from build123d import *

# Parameters (mm, degrees)
SKETCH1_R           = 13.000723037
SKETCH1_R_2         = 5.55
SKETCH1_R_3         = 0.8
PLACA_CABEZAL_DEPTH = 4
SKETCH2_W           = 7.5
SKETCH2_H           = 9
PATA_AL_HUESO_DEPTH = 4


with BuildPart() as part:
    # Sketch1 → Placa_cabezal (new body)
    with BuildSketch(Plane(origin=(0, -2, 0), x_dir=(1, 0, 0), z_dir=(0, 1, 0))):
        with Locations(Location((0, 0, 0), (0, 0, 270))):
            Circle(SKETCH1_R)
        with Locations(Location((0, 6.5, 0), (0, 0, 270))):
            Circle(SKETCH1_R_2, mode=Mode.SUBTRACT)
        with Locations(Location((-5.63, -3.25, 0), (0, 0, 270))):
            Circle(SKETCH1_R_2, mode=Mode.SUBTRACT)
        with Locations(Location((5.63, -3.25, 0), (0, 0, 270))):
            Circle(SKETCH1_R_2, mode=Mode.SUBTRACT)
        with Locations(Location((0, 0, 0), (0, 0, 270))):
            Circle(SKETCH1_R_3, mode=Mode.SUBTRACT)
    extrude(amount=PLACA_CABEZAL_DEPTH)

    # Sketch2 → Pata_al_hueso (add)
    with BuildSketch(Plane(origin=(0, -2, 0), x_dir=(1, 0, 0), z_dir=(0, 1, 0))):
        with Locations((-15.250723037, 0)):
            Rectangle(SKETCH2_W, SKETCH2_H)
    extrude(amount=PATA_AL_HUESO_DEPTH)


solid = part.part
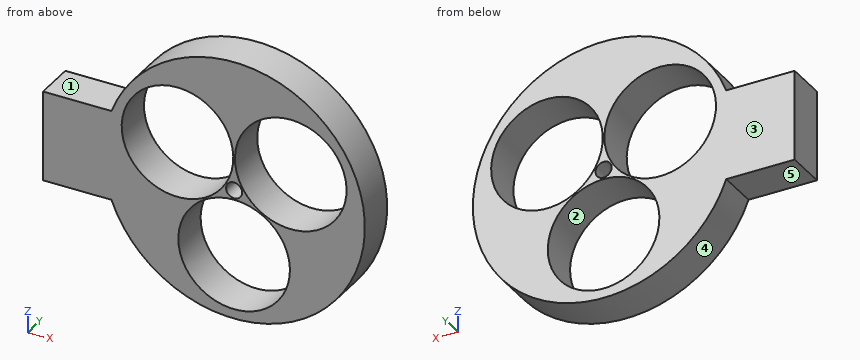
Here's how the part is built. I have some questions about the finished solid (model axes, mm). Face numbers are marked on the shaded views. A direction names the side the tool comes from. Round coordinates to 2 decimals unless told otherwise and drop trailing zeros. Order: outer loops, then holes, each group sorted by start corner. A loop starts at its lowest first (then second) coordinate and runs counter-clockwise, first axis right, second up. Notation, with made-up numbers: (62.5, -26.75) -> (88.5, -26.75) arc R17 ccw to (88.5, -4.75) -> close; hole circle Ø6 at (69.5, -1.75). An arc over 180 degrees is marked (long way). Return JSON: item names as keys, results as strings.
Q1. I need wall thicknesses on line 1 along X through (y, z) = (-0.6, 4); line 2 along X through (y, z) = (-0.9, 3.25); line 3 along Z through (x, y) = (-4.5, -1.2). Which ranges of each line are inside material? Lowest first, please. Write a range as from..to.
Filled sheet:
{"line 1": "x = -19..-11.13, -0.13..0.13, 11.13..12.37", "line 2": "x = -19..-11.18, -0.08..0.08, 11.18..12.59", "line 3": "z = -12.2..-9.75, -3.25..-2.18, 8.68..12.2"}
Q2. If we section it at C-C on y = -1.6: List the corners of the cut face in (x, z) for me.
Filled sheet:
{"outline": "(-19, -4.5) -> (-12.2, -4.5) arc R13 ccw (long way) to (-12.2, 4.5) -> (-19, 4.5) -> close; hole circle Ø11.1 at (-5.63, 3.25); hole circle Ø11.1 at (0, -6.5); hole circle Ø1.6 at (0, 0); hole circle Ø11.1 at (5.63, 3.25)"}
Q3. If we mould it in two halves opening along Z, with no side actions, what happens to the marked faces 1, 2 and 3? For each: released by +Z, released by -Z, zero draft, split by the parting line, or undercut.
Filled sheet:
{"face 1": "released by +Z", "face 2": "undercut", "face 3": "zero draft"}
Q4. If we section it at B-B on x = -2: List the corners of the cut face in (y, z) for me.
Filled sheet:
{"outline": "(-2, -12.85) -> (2, -12.85) -> (2, -11.68) -> (-2, -11.68) -> close; (-2, -1.32) -> (2, -1.32) -> (2, -0.95) -> (-2, -0.95) -> close; (-2, 7.45) -> (2, 7.45) -> (2, 12.85) -> (-2, 12.85) -> close"}
Q5. Which directions (+Z, -Z, +X, -X, +Y, -Y) give clear straight access to the entire face, cutting with the end or side of a thin tool? Please do the marked faces 4 and 5.
Filled sheet:
{"face 4": "+Y, -Y", "face 5": "-Z, -X, +Y, -Y"}
Q6. If we section it at D-D on z = -7: List the corners of the cut face in (x, y) for me, plus the area to 3 significant figures.
Filled sheet:
{"outline": "(-10.96, -2) -> (-5.53, -2) -> (-5.53, 2) -> (-10.96, 2) -> close; (5.53, -2) -> (10.96, -2) -> (10.96, 2) -> (5.53, 2) -> close", "area": "43.4 mm^2"}
Q7. If we section it at A-A on z = 2: List the corners of the cut face in (x, y) for me, plus the area to 3 significant figures.
Filled sheet:
{"outline": "(-19, -2) -> (-11.04, -2) -> (-11.04, 2) -> (-19, 2) -> close; (-0.22, -2) -> (0.22, -2) -> (0.22, 2) -> (-0.22, 2) -> close; (11.04, -2) -> (12.85, -2) -> (12.85, 2) -> (11.04, 2) -> close", "area": "40.9 mm^2"}
Q8. For pin 1 Ø1 at (y, z) = (-1.5, 2) entering from +X; pin 2 Ø1.2 at (x, y) = (-17, -0.5) entering from -Z; pin 3 Ø1.5 at (x, y) = (7, 0) entering from +Z, each with a flat end and sliding along its axis, tell me the tip position at first contact or that it passes through.
Filled sheet:
{"pin 1": "stops at x = 12.91", "pin 2": "stops at z = -4.5", "pin 3": "stops at z = 11.4"}
